Can you work these out from the model? Positions are in its coordinate system, mm. A direction names the side the tool comes from. Round coordinates to 2 decimals unless told otherwise and drop trailing zeros. Answer as CSV lines item,"result".
```python
from build123d import *

# Parameters (mm, degrees)
FILLET2_R           = 0.28575
CUT_EXTRUDE2_DEPTH  = 20.05
CIRPATTERN1_COUNT   = 16
SKETCH10_R          = 29.093421686
CUT_EXTRUDE3_DEPTH  = 15.24
SKETCH11_R          = 20.555223038
CUT_EXTRUDE4_DEPTH  = 10.16
SKETCH12_R          = 7.917123479
SKETCH12_R_2        = 4.826
BOSS_EXTRUDE1_DEPTH = 6.35
SKETCH_1_R          = 1.4351
CUT_EXTRUDE_1_DEPTH = 17.51


with BuildPart() as part:
    # Sketch4 → Revolve1 (revolve)
    with BuildSketch(Plane(origin=(0, 0, 0), x_dir=(0, 0, -1), z_dir=(1, 0, 0))):
        Polygon((-31.75, 6.35), (-31.75, 10.3251), (-19.05, 10.3251), (-19.05, 14.2875), (0, 14.2875), (0, 6.35), align=None)
    revolve(axis=Axis((0, 0, 19.05), (0, 0, 1)))

    # Fillet2
    fillet2_edges = [part.edges().sort_by_distance(p)[0] for p in [
        (0, -14.2875, 0),
        (0, -14.2875, 19.05),
        (0, -10.3251, 19.05),
        (0, -10.3251, 31.75),
    ]]
    fillet(fillet2_edges, radius=FILLET2_R)

    # Sketch7 → Cut-Extrude2 (cut, through all)
    with BuildSketch(Plane.XY.offset(19.05)):
        with BuildLine():
            ThreePointArc((-0.033120764, 10.318696845), (0, 10.31875), (0.033120764, 10.318696845))
            ThreePointArc((0.033120764, 10.318696845), (0.320422165, 10.413952701), (0.492309784, 10.663092059))
            ThreePointArc((0.492309784, 10.663092059), (1.160210792, 12.458856869), (2.090652449, 14.133712484))
            ThreePointArc((2.090652449, 14.133712484), (0, 14.2875), (-2.090652449, 14.133712484))
            ThreePointArc((-2.090652449, 14.133712484), (-1.160210792, 12.458856869), (-0.492309784, 10.663092059))
            ThreePointArc((-0.492309784, 10.663092059), (-0.320422165, 10.413952701), (-0.033120764, 10.318696845))
        make_face()
    cut_extrude2 = extrude(amount=-CUT_EXTRUDE2_DEPTH, mode=Mode.SUBTRACT)

    # CirPattern1: Cut-Extrude2 ×16 about axis
    cirpattern1_axis = Axis((0, 0, 0), (0, 0, 1))
    for i in range(1, CIRPATTERN1_COUNT):
        add(cut_extrude2.rotate(cirpattern1_axis, i * 360 / CIRPATTERN1_COUNT), mode=Mode.SUBTRACT)

    # Sketch10 → Cut-Extrude3 (cut)
    with BuildSketch(Plane.XY.offset(31.75)):
        Circle(SKETCH10_R)
    extrude(amount=-CUT_EXTRUDE3_DEPTH, mode=Mode.SUBTRACT)

    # Sketch11 → Cut-Extrude4 (cut)
    with BuildSketch(Plane(origin=(0, 0, 0), x_dir=(-1, 0, 0), z_dir=(0, 0, -1))):
        Circle(SKETCH11_R)
    extrude(amount=-CUT_EXTRUDE4_DEPTH, mode=Mode.SUBTRACT)

    # Sketch12 → Boss-Extrude1 (add)
    with BuildSketch(Plane.XY.offset(16.51)):
        Circle(SKETCH12_R)
        Circle(SKETCH12_R_2, mode=Mode.SUBTRACT)
    extrude(amount=-BOSS_EXTRUDE1_DEPTH)

    # Эскиз1 → Вырез-Вытянуть1 (cut, through all)
    with BuildSketch(Plane(origin=(0, 0, 0), x_dir=(-1, 0, 0), z_dir=(0, 0, -1))):
        with Locations((6.601034981, 4.40797498)):
            Circle(SKETCH_1_R)
        with Locations((4.40797498, -6.601034981)):
            Circle(SKETCH_1_R)
        with Locations((-6.601034981, -4.40797498)):
            Circle(SKETCH_1_R)
        with Locations((-4.40797498, 6.601034981)):
            Circle(SKETCH_1_R)
    extrude(amount=-CUT_EXTRUDE_1_DEPTH, mode=Mode.SUBTRACT)


solid = part.part
```
Q1. If I drill on line 1 along X through (y, z) = (10, 14.5); line 2 along Y through (x, z) = (-3.75, 15); line 3 along X through (y, z) = (-10.25, 11.5), over which ranges is the centre line in solid material (lowest first)? Write a range as [from, to].
Checks:
line 1,"[-8.12, -4.81], [-3.62, 3.62], [4.81, 8.12]"
line 2,"[-9.66, -7.88], [-5.33, -3.04], [3.04, 9.66]"
line 3,"[-8.2, -5.03], [-3.65, 3.65], [5.03, 8.2]"
Q2. On a 3-axis mill with a long thin cutter (end or side, diameter ignored), from which of +Z, -Z, +X, -X, +Y, -Y can I reach the whole of each face in a straight line? I mean faces 1 (the flat face through (0, -6, 10.16)), 2 (the cylindrical face through (11.981, -3.695, 13.379)), 3 (the cylindrical face through (-1.149, -12.434, 13.379)), 4 (the cylindrical face through (-5.859, 11.085, 13.379)), 5 (the cylindrical face through (11.085, 5.859, 13.379)). Say none if no direction works.
Checks:
face 1,"-Z, +X, -X, +Y, -Y"
face 2,"+Z, -Z"
face 3,"+Z, -Z, -Y"
face 4,"+Z, -Z, +Y"
face 5,"+Z, -Z, +X"
Q3. I'm going to push flat-ended pins straight in: pin 1 Ø3 at (y, z) = (0.5, 13.5) entering from +X; pin 2 Ø2 at (x, z) = (-4, 15.5) entering from +Y; pin 3 Ø1.5 at (x, z) = (-3, 11) entering from +Y. Where does each tip first touch, or does it pass through?
Checks:
pin 1,"x = 13.99"
pin 2,"y = 13.97"
pin 3,"y = 14.11"
Q4. We'd pull the mould along X, two halves only. Please class faces 6 (the cylindrical face through (11.928, 3.697, 13.379)), 7 (the cylindrical face through (-1.17, 12.48, 13.38)), 8 (the cylindrical face through (-14.015, -2.778, 13.291)), 9 (the flat face through (6, 0, 16.51)): pulls with the +X half, pulls with the -X half, needs draft (parallel to the pull), parting line crosses it, or undercut.
Checks:
face 6,"undercut"
face 7,"undercut"
face 8,"pulls with the -X half"
face 9,"needs draft"
Q5. Imagine slicing it at A-A (z = 14.25). Count the separate pieces of the cut face and the enclosed holes in it, then the cut area to 3 significant figures.
Checks:
separate pieces,"1"
enclosed holes,"5"
area,"400 mm²"
